Can you work these out from the model? Positions are in its coordinate system, mm. Face numbers are marked on the shaded views. Give positions to 0.01 mm unless a question says otherwise; leave off trailing zeros. Write each loop counter-clockwise with the first axis right and the second up, starting at its lowest first coordinate (ties: lowest second). Pieces come first, ordered by that corner, then holes.
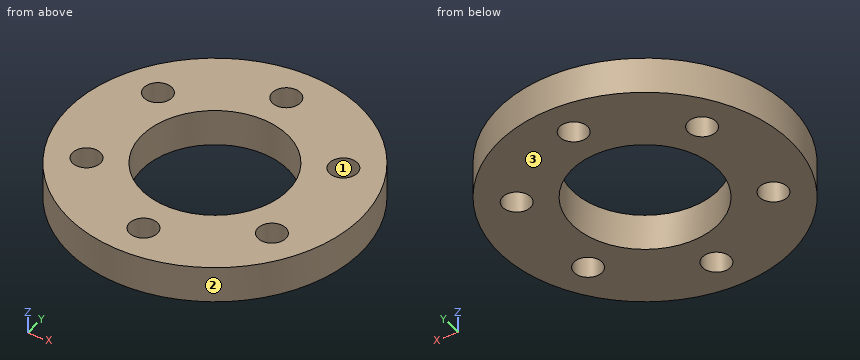
from build123d import *

# Parameters (mm, degrees)
SKETCH1_R           = 40
SKETCH1_R_2         = 20
BOSS_EXTRUDE1_DEPTH = 10
SKETCH2_R           = 3.831489411
CUT_EXTRUDE1_DEPTH  = 10
CIRPATTERN1_COUNT   = 6


with BuildPart() as part:
    # Sketch1 → Boss-Extrude1 (new body)
    with BuildSketch(Plane.XY):
        Circle(SKETCH1_R)
        Circle(SKETCH1_R_2, mode=Mode.SUBTRACT)
    extrude(amount=BOSS_EXTRUDE1_DEPTH)

    # Sketch2 → Cut-Extrude1 (cut)
    with BuildSketch(Plane.XY.offset(10)):
        with Locations((0, 29.911239538)):
            Circle(SKETCH2_R)
    cut_extrude1 = extrude(amount=-CUT_EXTRUDE1_DEPTH, mode=Mode.SUBTRACT)

    # CirPattern1: Cut-Extrude1 ×6 about axis
    cirpattern1_axis = Axis((0, 0, 0), (0, 0, 1))
    for i in range(1, CIRPATTERN1_COUNT):
        add(cut_extrude1.rotate(cirpattern1_axis, i * 360 / CIRPATTERN1_COUNT), mode=Mode.SUBTRACT)


solid = part.part
(1) Imagine slicing it at D-D, the plane x = -9. Write out the boundary of the cut face in (y, z).
Returned:
outline: (-38.97, 0) - (-17.86, 0) - (-17.86, 10) - (-38.97, 10) - close; (17.86, 0) - (38.97, 0) - (38.97, 10) - (17.86, 10) - close
(2) Imagine slicing it at B-B, the plane x = 0. Write out the boundary of the cut face in (y, z), plus the area to 3 significant figures.
Returned:
outline: (-40, 0) - (-33.74, 0) - (-33.74, 10) - (-40, 10) - close; (-26.08, 0) - (-20, 0) - (-20, 10) - (-26.08, 10) - close; (20, 0) - (26.08, 0) - (26.08, 10) - (20, 10) - close; (33.74, 0) - (40, 0) - (40, 10) - (33.74, 10) - close
area: 247 mm2
(3) Imagine slicing it at C-C, the plane z = 4. Write out the boundary of the cut face in (x, y), plus the area to 3 significant figures.
Returned:
outline: circle Ø80 at (0, 0); hole circle Ø7.66 at (-25.9, -14.96); hole circle Ø7.66 at (-25.9, 14.96); hole circle Ø40 at (0, 0); hole circle Ø7.66 at (0, -29.91); hole circle Ø7.66 at (0, 29.91); hole circle Ø7.66 at (25.9, -14.96); hole circle Ø7.66 at (25.9, 14.96)
area: 3,490 mm2
(4) If we mould it in two halves opening along X, with no side actions, what happens to the marked faces 1, 2 and 3? For each: +X half, -X half, draft (parallel to the pull), parting line (faces both ways), or undercut.
Returned:
face 1: undercut
face 2: parting line
face 3: draft
(5) Imagine slicing it at A-A, the plane y = 0. Write out the boundary of the cut face in (x, z), plus the area to 3 significant figures.
Returned:
outline: (-40, 0) - (-20, 0) - (-20, 10) - (-40, 10) - close; (20, 0) - (40, 0) - (40, 10) - (20, 10) - close
area: 400 mm2
(6) Will these pins go through, and if not, where does the flat tip stop? P1, Ø3, axis at x = 6, z = 2, coming from the -Y side; P2, Ø2, axis at x = -14, z = 2.5, coming from the -Y side; P3, Ø5, axis at y = -22.5, z = 2, coming from the +X side.
Returned:
P1: stops at y = -39.75
P2: stops at y = -37.83
P3: stops at x = 34.64
(7) If I drill on L1, parallel to Y at x = 0, z = 2; L2, parallel to Y at x = 29, z = 3.75; L3, parallel to X at y = -16, z = 6.75, over which ranges is the centre line in solid material (lowest first)?
Returned:
L1: y = -40 to -33.74, -26.08 to -20, 20 to 26.08, 33.74 to 40
L2: y = -27.55 to -17.21, -12.7 to 12.7, 17.21 to 27.55
L3: x = -36.66 to -29.59, -22.22 to -12, 12 to 22.22, 29.59 to 36.66
